Read the model definition and answer for the solid it produces. Units are mm, in the model's axes. A direction names the side the tool comes from. Coordinates: 2 decimals unless noted, no trailing zeros. Loops run counter-clockwise (first coordinate to the right, second up) from the corner with the lowest first, then second, coordinate; pieces in that order, holes last.
Q1. Flat-ended cylindrical pins translate along their axes: P1, Ø5, axis at x = 3.5, y = 25, coming from the +Z side (3 decimals); P2, Ø3, axis at x = 1, z = -21, coming from the +Y side; P3, Ø3, axis at x = -34, z = -14.5, coming from the +Y side. Find the tip coordinate at first contact, or state that the pin passes through.
Q2. Straight lines are drawn through the part: line 1 (X direction, y = 15.5, z = 3); line 2 (X direction, y = 25, z = 1); line 3 (Y direction, x = 33, z = -8). For each, find the intervals that lie inside material, in ascending order.
Q3. Section B-B (x = 32.5) is taken. Give the vertices of the cut face in (y, z) (3 decimals).
Q4. Which of the six approach directions +Z, -Z, +X, -X, +Y, -Y give full straight-line access (tool end or side, diameter ignored) to faces 4 (the face through (20.28, 23, 0)), 5 (the face through (14.27, 15, -21)), 6 (the face through (-16.416, 21.298, 17.559))?
Q5. Section A-A (y = 16) is taken. Give the vertices of the cut face in (x, z) (3 decimals).
Q6. The mould has two halves that part along X. Classify faces 1 (the face through (1, 12.5, 21)), 2 (the face through (-17.92, 21, 0)), 3 (the face through (1, 7, -22.145)): pulls with the +X half, pulls with the -X half, needs draft (parallel to the pull), parting line crosses it, or undercut.
Q7. Section C-C (y = 21) is taken. Give the vertices of the cut face in (x, z) (3 decimals).
Q8. Section D-D (x = -34) is taken. Give the vertices of the cut face in (y, z) (3 decimals).
from build123d import *

# Parameters (mm, degrees)
BOSS_EXTRUDE1_DEPTH = 31.42
BOSS_EXTRUDE2_DEPTH = 13.4
BOSS_EXTRUDE3_DEPTH = 17.6
SKETCH1_5_W         = 25.92
SKETCH1_5_H         = 3.16
SKETCH1_5_H_2       = 2.93
BOSS_EXTRUDE4_DEPTH = 12.5
FILLET2_SIZE        = 2


with BuildPart() as part:
    # Sketch1 → Boss-Extrude1 (new body)
    with BuildSketch(Plane(origin=(0, 0, 0), x_dir=(1, 0, 0), z_dir=(0, 1, 0))):
        with BuildLine():
            Line((-12.92, 19.215), (15.28, 19.215))
            ThreePointArc((15.28, 19.215), (18.815533906, 17.750533906), (20.28, 14.215))
            Line((20.28, 14.215), (20.28, -13.985))
            ThreePointArc((20.28, -13.985), (18.815533906, -17.520533906), (15.28, -18.985))
            Line((15.28, -18.985), (-12.92, -18.985))
            ThreePointArc((-12.92, -18.985), (-16.455533906, -17.520533906), (-17.92, -13.985))
            Line((-17.92, -13.985), (-17.92, 14.215))
            ThreePointArc((-17.92, 14.215), (-16.455533906, 17.750533906), (-12.92, 19.215))
        make_face()
    extrude(amount=BOSS_EXTRUDE1_DEPTH)

    # Sketch1<3> → Boss-Extrude2 (add)
    with BuildSketch(Plane(origin=(0, 0, 0), x_dir=(1, 0, 0), z_dir=(0, 1, 0))):
        with BuildLine():
            Line((-43.23, -22.145), (-11.65, -22.145))
            Line((-11.65, -22.145), (-11.65, -18.985))
            Line((-11.65, -18.985), (-12.92, -18.985))
            ThreePointArc((-12.92, -18.985), (-16.455533906, -17.520533906), (-17.92, -13.985))
            Line((-17.92, -13.985), (-17.92, 14.215))
            ThreePointArc((-17.92, 14.215), (-16.455533906, 17.750533906), (-12.92, 19.215))
            Line((-12.92, 19.215), (-11.65, 19.215))
            Line((-11.65, 19.215), (-11.65, 22.145))
            Line((-11.65, 22.145), (-43.23, 22.145))
            ThreePointArc((-43.23, 22.145), (-46.058427125, 20.973427125), (-47.23, 18.145))
            Line((-47.23, 18.145), (-47.23, -18.145))
            ThreePointArc((-47.23, -18.145), (-46.058427125, -20.973427125), (-43.23, -22.145))
        make_face()
    extrude(amount=BOSS_EXTRUDE2_DEPTH)

    # Sketch1<4> → Boss-Extrude3 (add)
    with BuildSketch(Plane(origin=(0, 0, 0), x_dir=(1, 0, 0), z_dir=(0, 1, 0))):
        with BuildLine():
            Line((14.27, -18.985), (14.27, -22.145))
            Line((14.27, -22.145), (43.23, -22.145))
            ThreePointArc((43.23, -22.145), (46.058427125, -20.973427125), (47.23, -18.145))
            Line((47.23, -18.145), (47.23, 18.145))
            ThreePointArc((47.23, 18.145), (46.058427125, 20.973427125), (43.23, 22.145))
            Line((43.23, 22.145), (14.27, 22.145))
            Line((14.27, 22.145), (14.27, 19.215))
            Line((14.27, 19.215), (15.28, 19.215))
            ThreePointArc((15.28, 19.215), (18.815533906, 17.750533906), (20.28, 14.215))
            Line((20.28, 14.215), (20.28, -13.985))
            ThreePointArc((20.28, -13.985), (18.815533906, -17.520533906), (15.28, -18.985))
            Line((15.28, -18.985), (14.27, -18.985))
        make_face()
    extrude(amount=BOSS_EXTRUDE3_DEPTH)

    # Sketch1<5> → Boss-Extrude4 (add)
    with BuildSketch(Plane(origin=(0, 0, 0), x_dir=(1, 0, 0), z_dir=(0, 1, 0))):
        with Locations((1.31, -20.565)):
            Rectangle(SKETCH1_5_W, SKETCH1_5_H)
        with Locations((1.31, 20.68)):
            Rectangle(SKETCH1_5_W, SKETCH1_5_H_2)
    extrude(amount=BOSS_EXTRUDE4_DEPTH)

    # Fillet2
    # a fillet whose section is not a circle: 2 mm, written as the material it takes off along each edge
    with BuildSketch(Plane(origin=(-17.92, 31.42, 13.985), x_dir=(0, -1, 0), z_dir=(0, 0, -1)), Plane(origin=(-12.92, 31.42, -19.215), x_dir=(0, -1, 0), z_dir=(1, 0, 0)), Plane(origin=(20.28, 31.42, -14.215), x_dir=(0, -1, 0), z_dir=(0, 0, 1)), Plane(origin=(15.28, 31.42, 18.985), x_dir=(0, -1, 0), z_dir=(-1, 0, 0))) as fillet2_piece_1:
        with BuildLine():
            Bezier((FILLET2_SIZE, 0), (0, 0), (0, -FILLET2_SIZE), weights=[1, 1, 1])
            Line((0, -FILLET2_SIZE), (0, 0))
            Line((0, 0), (FILLET2_SIZE, 0))
        make_face()
    extrude(amount=28.2, mode=Mode.SUBTRACT)
    with BuildSketch(Plane(origin=(-12.92, 31.42, -14.215), x_dir=(-1, 0, 0), z_dir=(0, 0, 1))) as fillet2_piece_2:
        with BuildLine():
            Bezier((5, FILLET2_SIZE), (5, 0), (5 - FILLET2_SIZE, 0), weights=[1, 1, 1])
            Line((5 - FILLET2_SIZE, 0), (5, 0))
            Line((5, 0), (5, FILLET2_SIZE))
        make_face()
    revolve(axis=Axis((-12.92, 31.42, -14.215), (0, -1, 0)), revolution_arc=90, mode=Mode.SUBTRACT)
    with BuildSketch(Plane(origin=(15.28, 31.42, -14.215), x_dir=(0, 0, -1), z_dir=(-1, 0, 0))) as fillet2_piece_3:
        with BuildLine():
            Bezier((5 - FILLET2_SIZE, 0), (5, 0), (5, FILLET2_SIZE), weights=[1, 1, 1])
            Line((5, FILLET2_SIZE), (5, 0))
            Line((5, 0), (5 - FILLET2_SIZE, 0))
        make_face()
    revolve(axis=Axis((15.28, 31.42, -14.215), (0, -1, 0)), revolution_arc=90, mode=Mode.SUBTRACT)
    with BuildSketch(Plane(origin=(15.28, 31.42, 13.985), x_dir=(1, 0, 0), z_dir=(0, 0, -1))) as fillet2_piece_4:
        with BuildLine():
            Bezier((5, FILLET2_SIZE), (5, 0), (5 - FILLET2_SIZE, 0), weights=[1, 1, 1])
            Line((5 - FILLET2_SIZE, 0), (5, 0))
            Line((5, 0), (5, FILLET2_SIZE))
        make_face()
    revolve(axis=Axis((15.28, 31.42, 13.985), (0, -1, 0)), revolution_arc=90, mode=Mode.SUBTRACT)
    with BuildSketch(Plane(origin=(-12.92, 31.42, 13.985), x_dir=(0, 0, 1), z_dir=(1, 0, 0))) as fillet2_piece_5:
        with BuildLine():
            Bezier((5, FILLET2_SIZE), (5, 0), (5 - FILLET2_SIZE, 0), weights=[1, 1, 1])
            Line((5 - FILLET2_SIZE, 0), (5, 0))
            Line((5, 0), (5, FILLET2_SIZE))
        make_face()
    revolve(axis=Axis((-12.92, 31.42, 13.985), (0, -1, 0)), revolution_arc=90, mode=Mode.SUBTRACT)


solid = part.part
Numbers:
1. P1: stops at z = 18.985
1. P2: stops at y = 12.5
1. P3: stops at y = 13.4
2. line 1: x = -17.92 to 47.23
2. line 2: x = -17.92 to 20.28
2. line 3: y = 0 to 17.6
3. outline: (0, -22.145) - (17.6, -22.145) - (17.6, 22.145) - (0, 22.145) - close
4. face 4: +Z, -Z, +X, +Y
4. face 5: -Z, +Y
4. face 6: +Z, -X, +Y
5. outline: (-17.92, -14.215) arc R5 ccw to (-12.92, -19.215) - (14.27, -19.215) - (14.27, -22.145) - (43.23, -22.145) arc R4 ccw to (47.23, -18.145) - (47.23, 18.145) arc R4 ccw to (43.23, 22.145) - (14.27, 22.145) - (14.27, 18.985) - (-12.92, 18.985) arc R5 ccw to (-17.92, 13.985) - close
6. face 1: undercut
6. face 2: pulls with the -X half
6. face 3: needs draft
7. outline: (-17.92, -14.215) arc R5 ccw to (-12.92, -19.215) - (15.28, -19.215) arc R5 ccw to (20.28, -14.215) - (20.28, 13.985) arc R5 ccw to (15.28, 18.985) - (-12.92, 18.985) arc R5 ccw to (-17.92, 13.985) - close
8. outline: (0, -22.145) - (13.4, -22.145) - (13.4, 22.145) - (0, 22.145) - close
